Geometry: see drawing. Coordinates: mm, zero at the bounding-box minimum. Round coordinates to 2 decimals unless told otherwise and drop trailing zeros. Write each loop counter-clockwise with the first axis right and the second up, starting at its lowest first coordinate (ties: lowest second). Pieces come first, ordered by that corner, then holes. Notation, with made-up numbers: (70, 2.25) -> (86, 2.25) arc R34 ccw to (86, 37.25) -> close; hole circle Ø7 at (82.25, 87.25). An arc over 180 degrees is marked (long way). Write item = value, one per line.
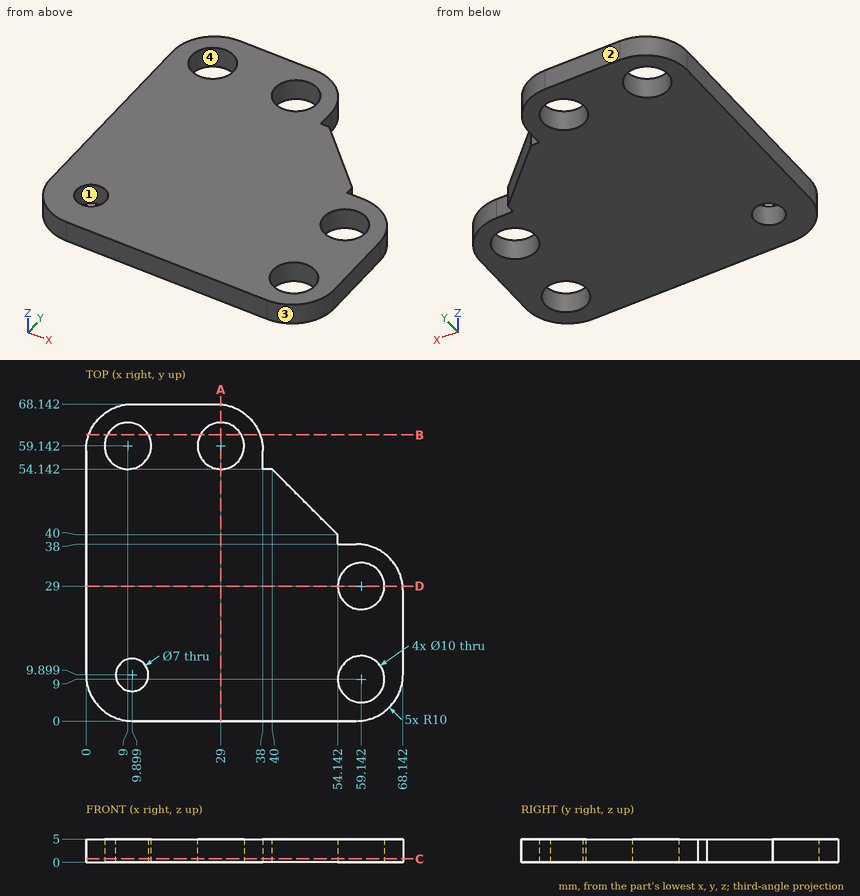
1) Cut plane B-B (y = 61.5). Return the cut outline in (x, z).
Solutions:
outline = (0.58, 0) -> (4.59, 0) -> (4.59, 5) -> (0.58, 5) -> close; (13.41, 0) -> (24.59, 0) -> (24.59, 5) -> (13.41, 5) -> close; (33.41, 0) -> (37.42, 0) -> (37.42, 5) -> (33.41, 5) -> close
2) Draft query along X for the marked faces 1, 2, 3 and 4. Return one class per face: +X half, -X half, draft (parallel to the pull), parting line (faces both ways), or undercut.
Solutions:
face_1 = undercut
face_2 = draft
face_3 = +X half
face_4 = undercut
3) Cut plane C-C (z = 0.75). Return the cut outline in (x, y).
Solutions:
outline = (0, 10) arc R10 ccw to (10, 0) -> (58.14, 0) arc R10 ccw to (68.14, 10) -> (68.14, 28) arc R10 ccw to (58.14, 38) -> (54.14, 38) -> (54.14, 40) -> (40, 54.14) -> (38, 54.14) -> (38, 58.14) arc R10 ccw to (28, 68.14) -> (10, 68.14) arc R10 ccw to (0, 58.14) -> close; hole circle Ø10 at (9, 59.14); hole circle Ø7 at (9.9, 9.9); hole circle Ø10 at (29, 59.14); hole circle Ø10 at (59.14, 9); hole circle Ø10 at (59.14, 29)
4) First-contact query: P1, Ø2, axis at x = 56.5, z = 2.5, coming from the +Y side; P2, Ø8, axis at x = 59.14, y = 29, coming from the +Z side; P3, Ø2, axis at y = 56, z = 3.5, coming from the +X side. Flat tips, straight axial feed; report the tip coordinate or a pass-through.
Solutions:
P1 = 38
P2 = through
P3 = 38
5) Cut plane A-A (x = 29). Return the cut outline in (y, z).
Solutions:
outline = (0, 0) -> (54.14, 0) -> (54.14, 5) -> (0, 5) -> close; (64.14, 0) -> (68.09, 0) -> (68.09, 5) -> (64.14, 5) -> close
6) Line query: L1, parallel to Y at x = 8.5, z = 3.1 (1 decimal); L2, parallel to Y at x = 9, z = 1.35; L3, parallel to X at y = 59.5, z = 0.8. Output: solid intervals per line, ascending. Write a range as from..to.
Solutions:
L1 = 0.1..6.7, 13.1..54.2, 64.1..68
L2 = 0.05..6.52, 13.28..54.14, 64.14..68.09
L3 = 0.09..4.01, 13.99..24.01, 33.99..37.91
